from build123d import *

# Parameters (mm, degrees)
F0_W      = 482.6
F0_H      = 857.25
F1_DEPTH  = 19.05
F3_D      = 8.001
F3_DEPTH  = 14.224
F3_TIP    = 2.4037429064
F5_D      = 15.0114
F5_DEPTH  = 14.224
F5_TIP    = 4.5098795482
F7_D      = 8.001
F7_DEPTH  = 25.4
F7_TIP    = 2.4037429064
F9_D      = 3.175
F9_DEPTH  = 14.224
F9_TIP    = 0.9538662327
F10_D     = 5.0038
F10_DEPTH = 14.224
F10_TIP   = 1.5032931827
F12_DEPTH = 25.4
F13_D     = 8.001
F13_DEPTH = 14.224
F13_TIP   = 2.4037429064


with BuildPart() as f1:
    # F0 (on Right) → F1 (new body)
    with BuildSketch(Plane.YZ):
        Rectangle(F0_W, F0_H)
    extrude(amount=F1_DEPTH)

    # F3
    with Locations(Plane.YZ.offset(19.05)):
        with Locations((-190.5, 419.1), (-9.525, 419.1), (171.45, 419.1), (231.775, 377.825), (231.775, 203.2), (231.775, -203.2), (231.775, -377.825), (171.45, -419.1), (-9.525, -419.1), (-190.5, -419.1)):
            Hole(F3_D / 2, depth=F3_DEPTH)
            with Locations((0, 0, -(F3_DEPTH + F3_TIP / 2))):  # 118° drill point
                Cone(0, F3_D / 2, F3_TIP, mode=Mode.SUBTRACT)

    # F5
    with Locations(Plane.YZ.offset(19.05)):
        with Locations((-217.424, 390.525)):
            Hole(F5_D / 2, depth=F5_DEPTH)
            with Locations((0, 0, -(F5_DEPTH + F5_TIP / 2))):  # 118° drill point
                Cone(0, F5_D / 2, F5_TIP, mode=Mode.SUBTRACT)

    # F7
    with Locations(Plane.XZ.offset(241.3)):
        with Locations((9.525, 390.525)):
            Hole(F7_D / 2, depth=F7_DEPTH)
            with Locations((0, 0, -(F7_DEPTH + F7_TIP / 2))):  # 118° drill point
                Cone(0, F7_D / 2, F7_TIP, mode=Mode.SUBTRACT)

    # F9
    with Locations(Plane.YZ.offset(19.05)):
        with Locations((-193.675, 301.625), (-87.376, 301.625), (104.775, 301.625), (104.775, 165.1), (9.525, 165.1), (-87.376, 165.1), (9.525, 301.625), (-193.675, 165.1)):
            Hole(F9_D / 2, depth=F9_DEPTH)
            with Locations((0, 0, -(F9_DEPTH + F9_TIP / 2))):  # 118° drill point
                Cone(0, F9_D / 2, F9_TIP, mode=Mode.SUBTRACT)

    # F10
    with Locations(Plane.YZ.offset(19.05)):
        with Locations((-204.724, -3.175), (-204.724, -34.925), (-204.724, -333.375), (-204.724, -365.125)):
            Hole(F10_D / 2, depth=F10_DEPTH)
            with Locations((0, 0, -(F10_DEPTH + F10_TIP / 2))):  # 118° drill point
                Cone(0, F10_D / 2, F10_TIP, mode=Mode.SUBTRACT)

    # F11 (on face) → F12 (cut)
    with BuildSketch(Plane.YZ.offset(19.05)):
        with BuildLine():
            ThreePointArc((207.9625, 365.125), (199.1281082875, 386.4531082875), (177.8, 395.2875))
            ThreePointArc((177.8, 395.2875), (156.4718917125, 343.7968917125), (207.9625, 365.125))
        make_face()
    extrude(amount=-F12_DEPTH, mode=Mode.SUBTRACT)

    # F13
    with Locations(Plane.YZ.offset(19.05)):
        with Locations((-190.5, 58.7375), (-9.525, 58.7375), (171.45, 58.7375)):
            Hole(F13_D / 2, depth=F13_DEPTH)
            with Locations((0, 0, -(F13_DEPTH + F13_TIP / 2))):  # 118° drill point
                Cone(0, F13_D / 2, F13_TIP, mode=Mode.SUBTRACT)


with BuildPart() as f14_1:
    # F14: instance of F1
    add(f1.part.mirror(Plane(origin=(9.525, 241.3, 0), x_dir=(-1, 0, 0), z_dir=(0, 1, 0))))


solid = f14_1.part
Verification items for the finished model (mm, model axes). Coordinates: 2 decimals unless noted, no trailing zeros. Answer as a JSON object with one key per item and string values. Group by question number.
Item 1: Mould release check, pull along Z, two halves, no side actions. Record for faces 1 (the flat face through (0, 486, 6)), 2 (the conical face through (1.1, 700.31, 389.25)), 3 (the flat face through (9, 486, 428.625)), 4 (the cylindrical face through (11.838, 692.526, 390.855)): +Z half, -Z half, draft (parallel to the pull), parting line (faces both ways), or undercut.
Item 2: Depth check by flat-ended pin: pin 1 (4.5 mm diameter, centred on y = 687.324, z = -3.175, fed in from +X); pin 2 (5 mm diameter, centred on y = 250.825, z = 203.2, fed in from +X). Enter the tip coordinate at first touch or a pass-through.
Item 3: Scan lines: probe 1 along Y at (x, z) = (15.5, 302); probe 2 along Y at (x, z) = (15.5, 203.2); probe 3 along Z at (x, y) = (11.75, 311.15) (1 decimal). Record each from-to range of solid material in increasing order.
Evaluation:
{
 "1": {"face 1": "draft", "face 2": "undercut", "face 3": "+Z half", "face 4": "undercut"},
 "2": {"pin 1": "stops at x = 4.67", "pin 2": "stops at x = 3.92"},
 "3": {"probe 1": "y = 241.3 to 376.28, 379.37 to 471.53, 474.62 to 568.43, 571.52 to 674.73, 677.82 to 723.9", "probe 2": "y = 241.3 to 246.82, 254.83 to 723.9", "probe 3": "z = -428.6 to -423.1, -415.1 to 54.7, 62.7 to 335.6, 394.6 to 415.1, 423.1 to 428.6"}
}
